Design review of the part built by this model. Coordinates are the model's own, in mm. Give positions to 0.01 mm unless a question says otherwise; leave off trailing zeros. Write each loop counter-clockwise with the first axis right and the second up, starting at its lowest first coordinate (ties: lowest second). Pieces come first, ordered by that corner, then holes. Notation, with made-up numbers: M -8.75,-2.75 L 15.25,-2.75 A16 cw 15.25,4.25 Z; hole C 21,31 d10. An arc over 180 degrees is marked long. Use a Markdown table: item, result. Add a question column.
```python
from build123d import *

# Parameters (mm, degrees)
SKETCH_1_W          = 8
SKETCH_1_H          = 4
SKETCH_2_R          = 2.1
CUT_EXTRUDE_1_DEPTH = 10


with BuildPart() as part:
    # 草图1 → 旋转1 (revolve)
    with BuildSketch(Plane.XY):
        with Locations((-43, 2)):
            Rectangle(SKETCH_1_W, SKETCH_1_H)
    revolve(axis=Axis((0, 0, 0), (0, 1, 0)))

    # 草图2 → 切除-拉伸1 (cut)
    with BuildSketch(Plane.XZ):
        with Locations((0, 42)):
            Circle(SKETCH_2_R)
        with Locations((29.69848481, 29.69848481)):
            Circle(SKETCH_2_R)
        with Locations((42, 0)):
            Circle(SKETCH_2_R)
        with Locations((29.69848481, -29.69848481)):
            Circle(SKETCH_2_R)
        with Locations((0, -42)):
            Circle(SKETCH_2_R)
        with Locations((-29.69848481, -29.69848481)):
            Circle(SKETCH_2_R)
        with Locations((-42, 0)):
            Circle(SKETCH_2_R)
        with Locations((-29.69848481, 29.69848481)):
            Circle(SKETCH_2_R)
    extrude(amount=-CUT_EXTRUDE_1_DEPTH, mode=Mode.SUBTRACT)


solid = part.part
```
(1) Add section C-C on z = -12. Give the boundary of the cut face in (x, y), then the cut area to 3 significant figures.
(2) The part is to be moulded in two halves that separate along Z. For faces 1 (the flat face through (11, 4, -38)), 2 (the cylindrical face through (-44.83, 2.03, 14.12)), 3 (the cylindrical face through (29.43, 1.97, 31.78)), say which applies: released by +Z, released by -Z, zero draft, split by the parting line, or undercut.
(3) Add section D-D on y = 2.3. Give the number of separate pieces and of enclosed holes in the cut face, then the cut area to 3 significant figures.
(4) Wall thickness on L1, parallel to Z at x = 0, y = 2.2; L2, parallel to X at y = 0.8, z = 30.5; L3, parallel to X at y = 1.65, z = 29: over which ranges is each line inside the solid? List them lowest first.
(5) Add section A-A on z = 0. Give the boundary of the cut face in (x, y), then the cut area to 3 significant figures.
(6) Add section B-B on x = -20.5. Give the boundary of the cut face in (y, z), then the cut area to 3 significant figures.
(7) For pin 1 (1.5 mm diameter, centred on x = 31, y = 2.5, fed in from +Z); pin 2 (6 mm diameter, centred on x = 16.5, z = 30, fed in from -Y), all flat-tipped, find the tip position at first contact; note any pin that passes through.
From the geometry:
| question | item | result |
|---|---|---|
| 1 | outline | M -45.44,0 L -37.11,0 L -37.11,4 L -45.44,4 Z; M 37.11,0 L 45.44,0 L 45.44,4 L 37.11,4 Z |
| 1 | area | 66.7 mm^2 |
| 2 | face 1 | zero draft |
| 2 | face 2 | split by the parting line |
| 2 | face 3 | undercut |
| 3 | separate pieces | 1 |
| 3 | enclosed holes | 9 |
| 3 | area | 2,050 mm^2 |
| 4 | L1 | z = -47 to -44.1, -39.9 to -39, 39 to 39.9, 44.1 to 47 |
| 4 | L2 | x = -35.76 to -31.64, -27.76 to -24.31, 24.31 to 27.76, 31.64 to 35.76 |
| 4 | L3 | x = -36.99 to -31.68, -27.72 to -26.08, 26.08 to 27.72, 31.68 to 36.99 |
| 5 | outline | M -47,0 L -44.1,0 L -44.1,4 L -47,4 Z; M -39.9,0 L -39,0 L -39,4 L -39.9,4 Z; M 39,0 L 39.9,0 L 39.9,4 L 39,4 Z; M 44.1,0 L 47,0 L 47,4 L 44.1,4 Z |
| 5 | area | 30.4 mm^2 |
| 6 | outline | M 0,-42.29 L 4,-42.29 L 4,-33.18 L 0,-33.18 Z; M 0,33.18 L 4,33.18 L 4,42.29 L 0,42.29 Z |
| 6 | area | 72.9 mm^2 |
| 7 | pin 1 | stops at z = 35.97 |
| 7 | pin 2 | passes through |
